```python
from build123d import *

# Parameters (mm, degrees)
F0_R      = 6.25
F1_DEPTH  = 11
F2_R      = 30
F3_DEPTH  = 25
F4_R      = 14
F4_R_2    = 10
F5_DEPTH  = 34
F5_FACE_R = 10
F6_DEPTH  = 25


with BuildPart() as f1:
    # F0 (on Top) → F1 (new body)
    with BuildSketch(Plane.XY):
        with BuildLine():
            Line((-49.861111, -11.516058), (-11.666667, -27.63854))
            ThreePointArc((-11.666667, -27.63854), (0, -30), (11.666667, -27.63854))
            Line((11.666667, -27.63854), (49.861111, -11.516058))
            ThreePointArc((49.861111, -11.516058), (57.5, 0), (49.861111, 11.516058))
            Line((49.861111, 11.516058), (11.666667, 27.63854))
            ThreePointArc((11.666667, 27.63854), (0, 30), (-11.666667, 27.63854))
            Line((-11.666667, 27.63854), (-49.861111, 11.516058))
            ThreePointArc((-49.861111, 11.516058), (-57.5, 0), (-49.861111, -11.516058))
        make_face()
        with Locations((-45, 0)):
            Circle(F0_R, mode=Mode.SUBTRACT)
        with Locations((45, 0)):
            Circle(F0_R, mode=Mode.SUBTRACT)
    extrude(amount=F1_DEPTH)

    # F2 (on Top) → F3 (join)
    with BuildSketch(Plane.XY):
        Circle(F2_R)
    extrude(amount=F3_DEPTH)

    # F4 (on Top) → F5 (join)
    with BuildSketch(Plane.XY):
        Circle(F4_R)
        Circle(F4_R_2, mode=Mode.SUBTRACT)
    extrude(amount=F5_DEPTH)

    # F5_face (on face) → F6 (cut)
    with BuildSketch(Plane.XY.offset(25)):
        Circle(F5_FACE_R)
    extrude(amount=-F6_DEPTH, mode=Mode.SUBTRACT)


solid = f1.part
```
Geometry: final body of the model. Coordinates: model frame, mm. A direction names the side the tool comes from. Give positions to 0.01 mm unless a question says otherwise; leave off trailing zeros. Order: outer loops, then holes, each group sorted by start corner. A loop starts at its lowest first (then second) coordinate and runs counter-clockwise, first axis right, second up. Notation, with made-up numbers: (48.25, -12.75) -> (75.25, -12.75) arc R24 cw to (75.25, 6.25) -> close; hole circle Ø6 at (45.25, 0). An arc over 180 degrees is marked (long way). Write each question's results on one line, items separated by ' | '. Start each with the question number.
1) First-contact query: pin 1 (2 mm diameter, centred on x = -28.5, y = 9, fed in from -Z); pin 2 (10 mm diameter, centred on y = 7.5, z = 21, fed in from -X); pin 3 (11 mm diameter, centred on x = 45, y = 0, fed in from -Z); pin 4 (8 mm diameter, centred on x = 24.5, z = 11.5, fed in from -Y). Flat tips, straight axial feed; report the tip coordinate or a pass-through.
2) Section C-C (z = 5.5). Return loops of the section in (x, y), then the cut area to 3 significant figures.
3) Section A-A (x = 0). Return loops of the section in (y, z), then the cut area to 3 significant figures.
4) Draft query along X for faces 3 (the cylindrical face through (-2.17, -9.76, 17.24)), 4 (the cylindrical face through (-39.04, 1.88, 5.42)), 5 (the flat face through (12, 0, 0)), 6 (the flat face through (31.031, 19.464, 5.423)). Return one class per face: pulls with the +X half, pulls with the -X half, needs draft (parallel to the pull), parting line crosses it, or undercut.
5) Section D-D (x = 18). Return loops of the section in (y, z).
6) Line query: line 1 (Y direction, x = 0, z = 12); line 2 (Z direction, x = -2, y = -16); line 3 (Z direction, x = 30, y = 8). Output: solid intervals per line, ascending. Write a range as from..to.
7) Set-up query: faces 1 (the cylindrical face through (-57.5, 0.2, 5.4)), 2 (the cylindrical face through (12.932, -5.362, 29.437)). Return all of +Z, -Z, +X, -X, +Y, -Y with unobstructed straight access to the full face (end or side cutting, diameter ignored); none if empty.
8) Section B-B (y = 0). Return loops of the section in (x, z), then the cut area to 3 significant figures.
Calculated:
1) pin 1: z = 0 | pin 2: x = -29.9 | pin 3: through | pin 4: y = -23.9
2) outline: (-49.86, -11.52) -> (-11.67, -27.64) arc R30 ccw to (11.67, -27.64) -> (49.86, -11.52) arc R12.5 ccw to (49.86, 11.52) -> (11.67, 27.64) arc R30 ccw to (-11.67, 27.64) -> (-49.86, 11.52) arc R12.5 ccw to start; hole circle Ø12.5 at (-45, 0); hole circle Ø20 at (0, 0); hole circle Ø12.5 at (45, 0) | area: 4,050 mm2
3) outline: (-30, 0) -> (-10, 0) -> (-10, 34) -> (-14, 34) -> (-14, 25) -> (-30, 25) -> close; (10, 0) -> (30, 0) -> (30, 25) -> (14, 25) -> (14, 34) -> (10, 34) -> close | area: 1,070 mm2
4) face 3: undercut | face 4: undercut | face 5: needs draft | face 6: pulls with the +X half
5) outline: (-24.97, 0) -> (24.97, 0) -> (24.97, 11) -> (24, 11) -> (24, 25) -> (-24, 25) -> (-24, 11) -> (-24.97, 11) -> close
6) line 1: -30..-10, 10..30 | line 2: 0..25 | line 3: 0..11
7) face 1: +Z, -Z, -X | face 2: +Z
8) outline: (-57.5, 0) -> (-51.25, 0) -> (-51.25, 11) -> (-57.5, 11) -> close; (-38.75, 0) -> (-10, 0) -> (-10, 34) -> (-14, 34) -> (-14, 25) -> (-30, 25) -> (-30, 11) -> (-38.75, 11) -> close; (10, 0) -> (38.75, 0) -> (38.75, 11) -> (30, 11) -> (30, 25) -> (14, 25) -> (14, 34) -> (10, 34) -> close; (51.25, 0) -> (57.5, 0) -> (57.5, 11) -> (51.25, 11) -> close | area: 1,400 mm2
